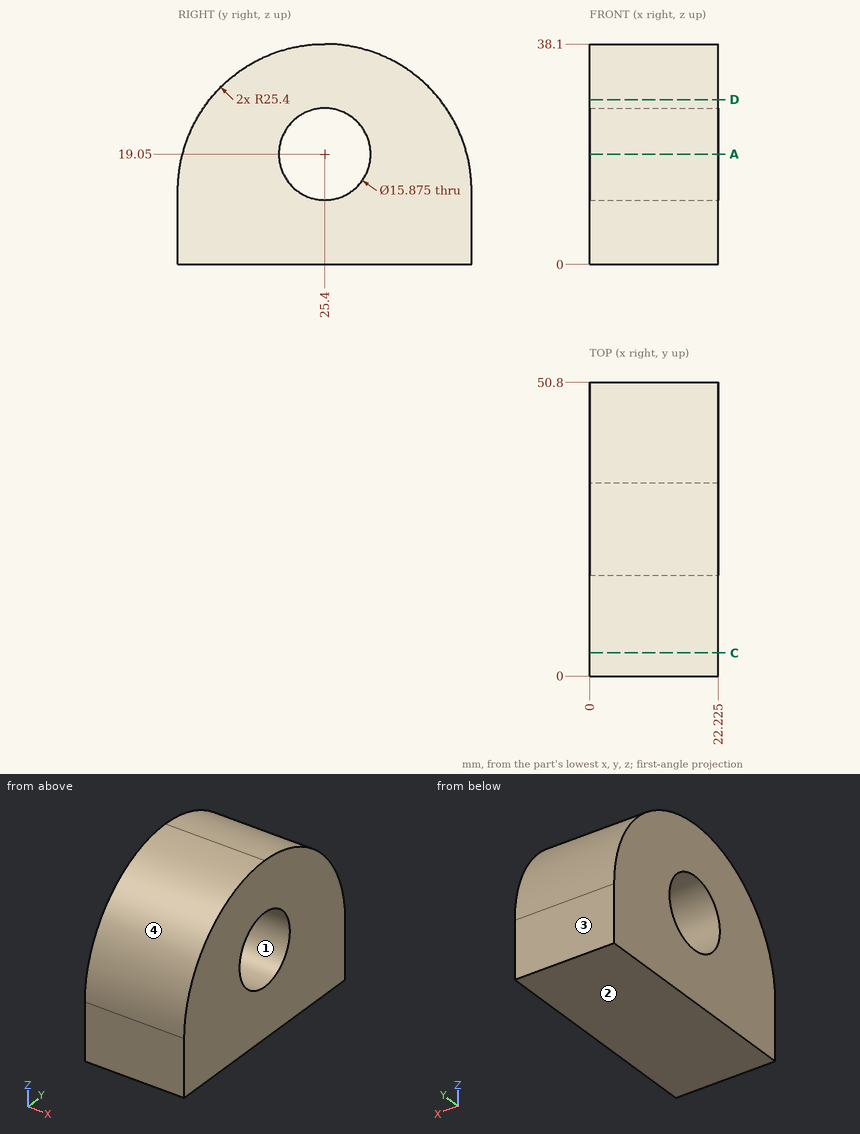
Part print with two shaded views. Sizes in mm from the minimum x, y, z corner. Coordinates: 2 decimals unless noted, no trailing zeros. Write each loop counter-clockwise with the first axis right and the second up, starting at its lowest first coordinate (ties: lowest second). Pieces come first, ordered by that corner, then holes. Notation, with made-up numbers: (40.25, 83) -> (99.25, 83) arc R7 cw to (99.25, 95) -> close; hole circle Ø4 at (71, 5). An arc over 180 degrees is marked (long way). Return JSON: item names as keys, results as strings. Group by question number.
Q1. Cut at D-D, the plane z = 28.5. Give the cut face in (x, y) (3 decimals), then the cut area to 3 significant figures.
Q2. Pull direction Z, two halves, no side cores. Call the marked faces 1, 2, 3 and 4: released by +Z, released by -Z, zero draft, split by the parting line, or undercut.
Q3. Cut at C-C, the plane y = 4. Give the cut face in (x, z) (3 decimals), then the cut area to 3 significant figures.
Q4. Flat gauge pin, fed straight in: pin 1 (1.5 mm diameter, centred on x = 8, z = 26.5, fed in from -Y). Where does the tip first touch, or does it go through?
Q5. Drill centre lines: line 1 (Z direction, x = 10.25, y = 25.4); line 2 (Z direction, x = 6.75, y = 20); line 3 (Y direction, x = 2.75, z = 17). Where is each one in solid material? Low to high.
Q6. Cut at A-A, the plane z = 19.05. Give the cut face in (x, y) (1 decimal), then the cut area to 3 significant figures.
Returned:
{
 "1": {"outline": "(0, 5.512) -> (22.225, 5.512) -> (22.225, 45.288) -> (0, 45.288) -> close", "area": "884 mm2"},
 "2": {"face 1": "undercut", "face 2": "released by -Z", "face 3": "zero draft", "face 4": "released by +Z"},
 "3": {"outline": "(0, 0) -> (22.225, 0) -> (22.225, 26.382) -> (0, 26.382) -> close", "area": "586 mm2"},
 "4": {"pin 1": "stops at y = 3.61"},
 "5": {"line 1": "z = 0 to 11.11, 26.99 to 38.1", "line 2": "z = 0 to 13.23, 24.87 to 37.52", "line 3": "y = 0.37 to 17.73, 33.07 to 50.43"},
 "6": {"outline": "(0, 0.8) -> (22.2, 0.8) -> (22.2, 17.5) -> (0, 17.5) -> close; (0, 33.3) -> (22.2, 33.3) -> (22.2, 50) -> (0, 50) -> close", "area": "740 mm2"}
}
